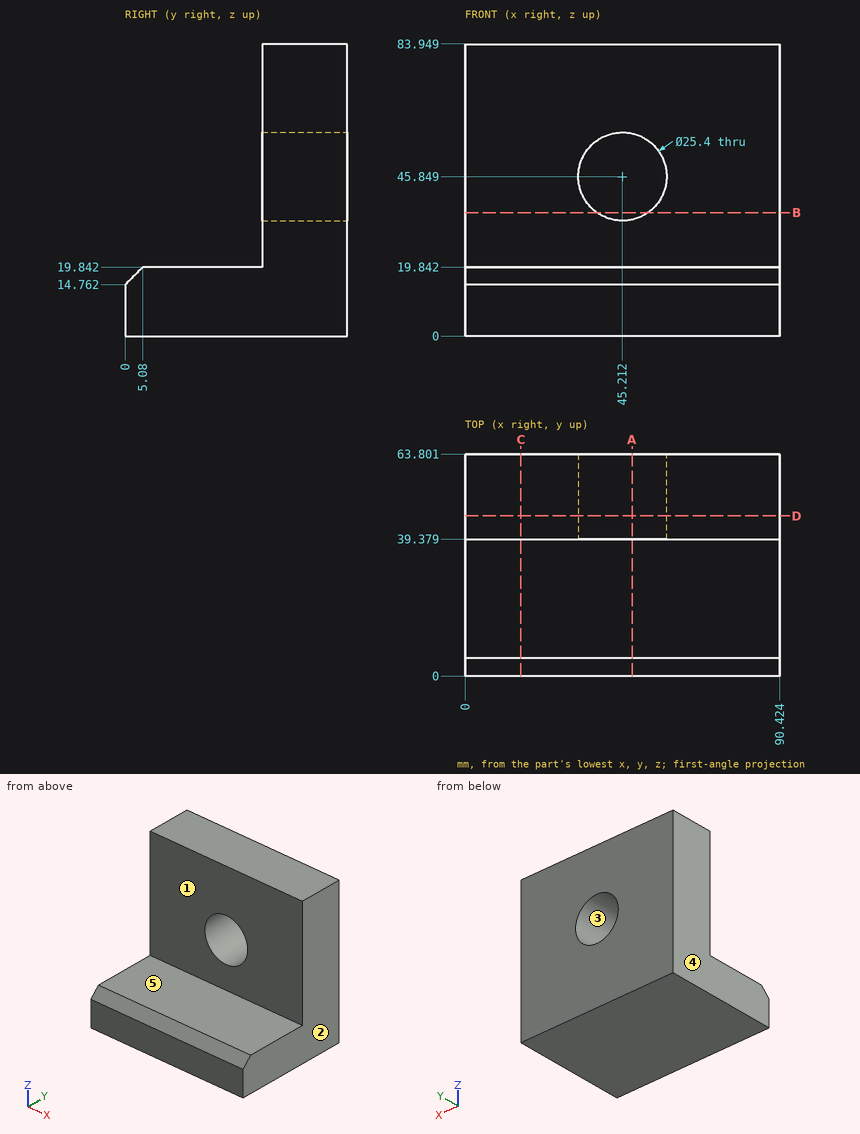
Part print with two shaded views. Sizes in mm from the minimum x, y, z corner. A direction names the side the tool comes from. Round coordinates to 2 decimals unless told otherwise and drop trailing zeros. Write each loop counter-clockwise with the first axis right and the second up, starting at its lowest first coordinate (ties: lowest second). Pieces come first, ordered by that corner, then holes. Notation, with made-up numbers: M -18,49 L 27,49 A31 cw 27,74 Z; hole C -11.75,-1 d2. An arc over 180 degrees is marked long. Put each result on its own line as item: value. Start each with the question number.
1) 3-axis set-ups, long thin cutter, end or side, ignore diameter. For the marked faces 1 and 2: which of +Z, -Z, +X, -X, +Y, -Y reach the whole face in a straight line?
2) Drill centre lines: probe 1 along Y at (x, z) = (83, 67.5); probe 2 along Z at (x, y) = (7.5, 22); probe 3 along X at (y, z) = (53, 47.5) (1 decimal). Where is each one in solid material? Low to high. Write a range as [from, to].
3) Saw through at B-B, the plane z = 35.5. Write the cut outline in (x, y).
4) Saw through at A-A, the plane x = 48. Write the cut outline in (y, z).
5) Pull direction X, two halves, no side cores. Call the marked faces 3, 4 and 5: pulls with the +X half, pulls with the -X half, needs draft (parallel to the pull), parting line crosses it, or undercut.
6) Pin check, flat tip, straight feed: pin 1 Ø8 at (x, z) = (14, 43) entering from -Y. Stop position of the tip, or through.
7) Saw through at D-D, the plane y = 46. Write the cut outline in (x, z).
8) Saw through at C-C, the plane x = 16. Write the cut outline in (y, z).
Resolved:
1. face 1: +Z, +X, -X, -Y
1. face 2: +Z, -Z, +X, +Y, -Y
2. probe 1: [39.38, 63.8]
2. probe 2: [0, 19.84]
2. probe 3: [0, 32.6], [57.8, 90.4]
3. outline: M 0,39.38 L 37.85,39.38 L 37.85,63.8 L 0,63.8 Z; M 52.57,39.38 L 90.42,39.38 L 90.42,63.8 L 52.57,63.8 Z
4. outline: M 0,0 L 63.8,0 L 63.8,33.46 L 39.38,33.46 L 39.38,19.84 L 5.08,19.84 L 0,14.76 Z; M 39.38,58.24 L 63.8,58.24 L 63.8,83.95 L 39.38,83.95 Z
5. face 3: undercut
5. face 4: pulls with the -X half
5. face 5: needs draft
6. pin 1: y = 39.38
7. outline: M 0,0 L 90.42,0 L 90.42,83.95 L 0,83.95 Z; hole C 45.21,45.85 d25.4
8. outline: M 0,0 L 63.8,0 L 63.8,83.95 L 39.38,83.95 L 39.38,19.84 L 5.08,19.84 L 0,14.76 Z
